Autodesk Inventor part; units mm, degrees
ref_plane "YZ Plane" through (0, 0, 0) normal (1, 0, 0) x (0, 1, 0)
ref_plane "XZ Plane" through (0, 0, 0) normal (0, 1, 0) x (-1, 0, 0)
ref_plane "XY Plane" through (0, 0, 0) normal (0, 0, 1) x (1, 0, 0)
sketch "Sketch3" plane through (0, 0, 0) normal (1, 0, 0) x (0, 1, 0)
  line L0 (25, -26.5) -> (-25, -26.5)
  line L1 (-25, -26.5) -> (-25, 26.5)
  line L2 (-25, 26.5) -> (25, 26.5)
  line L3 (25, 26.5) -> (25, -26.5)
  line L4 (25, -26.5) -> (-25, 26.5) construction
  line L5 (-25, -26.5) -> (25, 26.5) construction
  line L6 (25, 26.5) -> (10, 26.5)
  line L7 (10, 26.5) -> (10, 16.5)
  line L8 (10, 16.5) -> (-10, 16.5)
  line L9 (-10, 16.5) -> (-10, 26.5)
  line L10 (-10, 26.5) -> (-25, 26.5)
  line L11 (25, -26.5) -> (10, -26.5)
  line L12 (10, -26.5) -> (10, -16.5)
  line L13 (10, -16.5) -> (-10, -16.5)
  line L14 (-10, -16.5) -> (-10, -26.5)
  line L15 (-10, -26.5) -> (-25, -26.5)
  point P0 (0, 0)
  dimension "d0" = 50
  dimension "d1" = 53
  dimension "d2" = 15
  dimension "d3" = 10
  dimension "d4" = 20
  dimension "d5" = 10
  dimension "d6" = 15
  dimension "d7" = 10
  dimension "d8" = 20
  dimension "d9" = 10
  dimension "d10" = 15
extrude "Extrusion1" add sketch "Sketch3" along normal blind 10 contours L0 L12 L13 L14 L1 L2 L9 L8 L7 L3
sketch "Sketch5" plane through (10, 0, 0) normal (1, 0, 0) x (0, 0, -1)
  circle A0 centre (0, 0) radius 7.5
  circle A1 centre (0, 0) radius 5
  dimension "d13" = 15
  dimension "d33" = 10
sketch "Sketch6" plane through (0, -25, -26.5) normal (0, -1, 0) x (1, 0, 0)
  circle A0 centre (5, 26.5) radius 1.25
  dimension "d30" = 2.5
extrude "Extrusion2" cut sketch "Sketch5" against normal blind 10 contours A0 | A1
extrude "Extrusion3" cut sketch "Sketch6" against normal blind 10
extrude "Extrusion4" add sketch "Sketch5" against normal blind 2
fillet "Fillet1" radius 2 1 edges at (0, 0, 7.5)
properties part number "prepazka_kola"
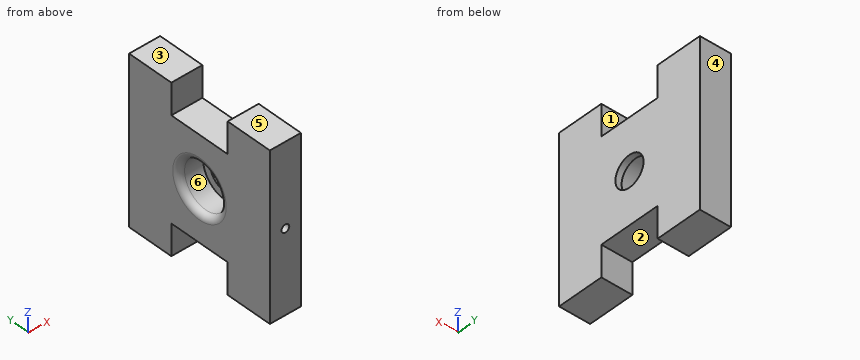
Design review of the part built by this model. Coordinates are the model's own, in mm. Face numbers are marked on the shaded views. A direction names the side the tool comes from. Coordinates: 2 decimals unless noted, no trailing zeros. Order: outer loops, then holes, each group sorted by start corner. A loop starts at its lowest first (then second) coordinate and runs counter-clockwise, first axis right, second up. Notation, with made-up numbers: M -33.75,-4 L -25.75,-4 A15 ccw -25.75,20 Z; hole C 46.25,5.25 d6. An arc over 180 degrees is marked long. Answer as a JSON object with one key per item and string values. Group by question number.
1) Add section C-C, the plane x = 2.75. Write out the cut boundary in (y, z), then the cut area to 3 significant figures.
2) Add section D-D, the plane z = 0. Write out the cut boundary in (x, y), then the cut area to 3 significant figures.
3) For pin 1 (4 mm diameter, centred on x = 7, y = 3.5, fed in from +Z); pin 2 (5 mm diameter, centred on x = 6.5, y = 3, fed in from -Z), all flat-tipped, find the tip position at first contact; note any pin that passes through.
4) Wall thickness on L1, parallel to Y at x = 6.5, z = -22; L2, parallel to Y at x = 9.05, z = 0; L3, parallel to Z at x = 1, y = -8: over which ranges is each line inside the solid? List them lowest first.
5) Add section B-B, the plane z = 20.5. Write out the cut boundary in (x, y).
6) Mouldability with a two-part tool opening along Y and no side actions: class the marked faces 4, 5 and 6 as pulls with the +Y half, pulls with the -Y half, needs draft (parallel to the pull), parting line crosses it, or undercut.
7) Add section A-A, the plane y = 0. Write out the cut boundary in (x, z), then the cut area to 3 significant figures.
8) Tool access review of the marked faces 1, 2 and 3: name each direction out of +Z, -Z, +X, -X, +Y, -Y from which nothing blocks a thin tool from reaching the whole face with its end or side.
Computed values:
{
 "1": {"outline": "M -25,-26.5 L -10,-26.5 L -10,-16.5 L 10,-16.5 L 10,-26.5 L 25,-26.5 L 25,26.5 L 10,26.5 L 10,16.5 L -10,16.5 L -10,26.5 L -25,26.5 Z; hole C 0,0 d15", "area": "2,070 mm^2"},
 "2": {"outline": "M 0,-25 L 3.75,-25 L 3.75,-15 L 6.25,-15 L 6.25,-25 L 10,-25 L 10,-5 L 8,-5 L 8,-7.5 L 2,-7.5 A2 ccw 0,-9.5 Z; M 0,9.5 A2 ccw 2,7.5 L 8,7.5 L 8,5 L 10,5 L 10,25 L 0,25 Z", "area": "333 mm^2"},
 "3": {"pin 1": "stops at z = 16.5", "pin 2": "stops at z = -16.5"},
 "4": {"L1": "y = -25 to -10, 10 to 25", "L2": "y = -25 to -5, 5 to 25", "L3": "z = -16.5 to 16.5"},
 "5": {"outline": "M 0,-25 L 10,-25 L 10,-10 L 0,-10 Z; M 0,10 L 10,10 L 10,25 L 0,25 Z"},
 "6": {"face 4": "pulls with the +Y half", "face 5": "needs draft", "face 6": "undercut"},
 "7": {"outline": "M 0,-16.5 L 10,-16.5 L 10,-5 L 8,-5 L 8,-7.5 L 2,-7.5 A2 ccw 0,-9.5 Z; M 0,9.5 A2 ccw 2,7.5 L 8,7.5 L 8,5 L 10,5 L 10,16.5 L 0,16.5 Z", "area": "188 mm^2"},
 "8": {"face 1": "+Z, +X, -X", "face 2": "-Z, +X, -X", "face 3": "+Z, +X, -X, +Y, -Y"}
}
